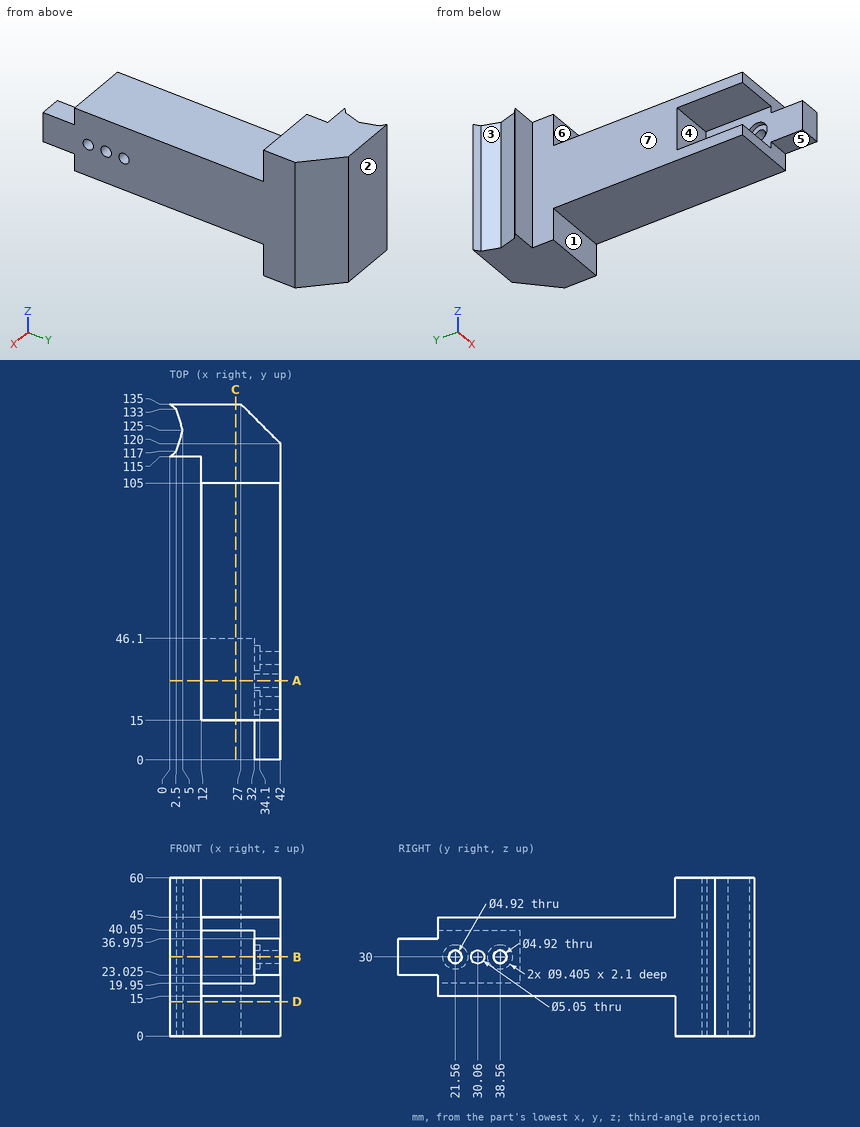
Geometry check sheet. Reference: drawing and pictorial views, mm from the part's lowest x, y, z. A direction names the side the tool comes from. Round coordinates to 2 decimals unless told otherwise and drop trailing zeros. Write each loop counter-clockwise with the first axis right and the second up, starting at its lowest first coordinate (ties: lowest second). Pieces come first, ordered by that corner, then holes.
1. Section check B-B on z = 30. State how many separate pieces and enclosed holes the cut face has, plus the area to 3 significant figures.
2. Gauge pin test, flat ends, axial feed: P1, Ø12, axis at x = 34.5, z = 10, coming from the -Y side; P2, Ø15, axis at y = 21.56, z = 30, coming from the -X side; P3, Ø3, axis at x = 27.5, y = 41, coming from the -Z side; P4, Ø5, axis at x = 8, y = 32.5, coming from the +Z side. Record the tip position at first contact, or that the pin passes through.
3. Section check D-D on z = 13. Enter the section's corners in (x, y), plus the area to 4 significant figures.
4. Access from +Z, -Z, +X, -X, +Y, -Y to the whole of each face (thin tool, end or side, straight path). Record for the marked faces 4, 5, 6 and 7.
5. Scan lines: L1, parallel to Y at x = 37, z = 30 (3 decimals); L2, parallel to Y at x = 36.25, z = 30 (3 decimals); L3, parallel to Z at x = 39.5, y = 21.56. Record each from-to range of solid material in increasing order.
6. Section check C-C on x = 25. Enter the section's corners in (y, z), plus the area to 3 significant figures.
7. Section check A-A on y = 30.06. Enter the section's corners in (x, z) (3 decimals), plus the area to 4 significant figures.
8. Draft check along Y on the marked faces 1, 2 and 3. Enter one of: +Y half, -Y half, draft (parallel to the pull), parting line (faces both ways), or undercut.
Answer:
1. separate pieces: 4
1. enclosed holes: 0
1. area: 3,020 mm2
2. P1: stops at y = 15
2. P2: stops at x = 32
2. P3: stops at z = 15
2. P4: passes through
3. outline: (0, 115) - (12, 115) - (12, 105) - (42, 105) - (42, 120) - (27, 135) - (0, 135) - (2.5, 133) - (5, 125) - (2.5, 117) - close
3. area: 962.5 mm2
4. face 4: -X, -Y
4. face 5: -Z, +X, -X, -Y
4. face 6: +Z, +X, -X, -Y
4. face 7: +Z, -Z, -X, -Y
5. L1: y = 0 to 19.1, 24.02 to 27.535, 32.585 to 36.1, 41.02 to 125
5. L2: y = 0 to 19.1, 24.02 to 27.535, 32.585 to 36.1, 41.02 to 125.75
5. L3: z = 15 to 27.54, 32.46 to 45
6. outline: (15, 15) - (105, 15) - (105, 0) - (135, 0) - (135, 60) - (105, 60) - (105, 45) - (15, 45) - (15, 40.05) - (46.1, 40.05) - (46.1, 19.95) - (15, 19.95) - close
6. area: 3,870 mm2
7. outline: (12, 15) - (42, 15) - (42, 27.475) - (32, 27.475) - (32, 19.95) - (12, 19.95) - close; (12, 40.05) - (32, 40.05) - (32, 32.525) - (42, 32.525) - (42, 45) - (12, 45) - close
7. area: 447.5 mm2
8. face 1: -Y half
8. face 2: +Y half
8. face 3: undercut
